```python
from build123d import *

# Parameters (mm, degrees)
SKETCH1_R           = 6.25
BOSS_EXTRUDE1_DEPTH = 4
BOSS_EXTRUDE5_START = -8
SKETCH7_R           = 8.125
SKETCH7_R_2         = 6.125
BOSS_EXTRUDE5_DEPTH = 12


with BuildPart() as part:
    # Sketch1 → Boss-Extrude1 (new body)
    with BuildSketch(Plane.XY):
        with BuildLine():
            Line((85.864132579, -9.289310318), (33.098166031, -56.8))
            Line((33.098166031, -56.8), (-33.098166031, -56.8))
            Line((-33.098166031, -56.8), (-85.864132579, -9.289310318))
            ThreePointArc((-85.864132579, -9.289310318), (-77.904361198, 12.493457969), (-68.552689408, -8.729011007))
            Line((-68.552689408, -8.729011007), (-28.491797611, -44.8))
            Line((-28.491797611, -44.8), (28.491797611, -44.8))
            Line((28.491797611, -44.8), (68.552689408, -8.729011007))
            ThreePointArc((68.552689408, -8.729011007), (77.904361198, 12.493457969), (85.864132579, -9.289310318))
        make_face()
        with Locations((-77.5, 0)):
            Circle(SKETCH1_R, mode=Mode.SUBTRACT)
        with Locations((77.5, 0)):
            Circle(SKETCH1_R, mode=Mode.SUBTRACT)
    extrude(amount=BOSS_EXTRUDE1_DEPTH)

    # Sketch7 → Boss-Extrude5 (add)
    with BuildSketch(Plane.XY.offset(4).offset(BOSS_EXTRUDE5_START)):
        with Locations((-77.5, 0)):
            Circle(SKETCH7_R)
        with Locations((-77.5, 0)):
            Circle(SKETCH7_R_2, mode=Mode.SUBTRACT)
    boss_extrude5 = extrude(amount=BOSS_EXTRUDE5_DEPTH)

    # Mirror1: Boss-Extrude5 across plane
    add(boss_extrude5.mirror(Plane(origin=(0, 0, 0), x_dir=(0, 0, 1), z_dir=(1, 0, 0))))


solid = part.part
```
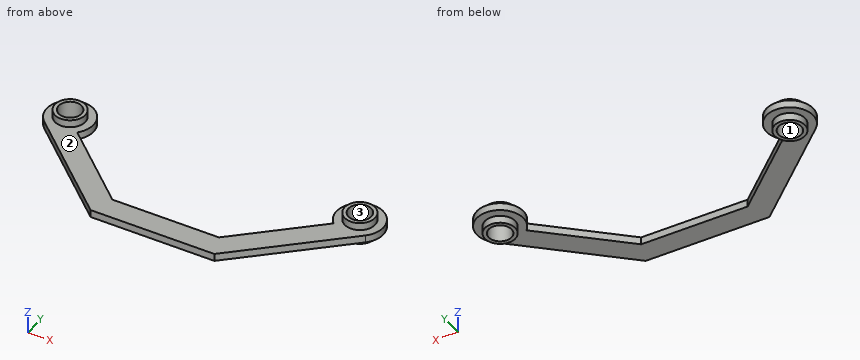
Model file for the job. Use its own axes, mm. Face numbers are marked on the shaded views. Coordinates: 2 decimals unless noted, no trailing zeros. Loops run counter-clockwise (first coordinate to the right, second up) from the corner with the lowest first, then second, coordinate; pieces in that order, holes last. Notation, with made-up numbers: (-11, -1) - (45, -1) arc R26 ccw to (45, 19) - close; hole circle Ø8 at (-36, -24.5). An arc over 180 degrees is marked (long way). Answer as a JSON object with one key per item and string values. Group by question number.
(1) Cut at B-B (y = -21.5). Give the cut face in (x, z), then the cut area to 3 significant figures.
(2) Cut at A-A (y = 0). State how many separate pieces and enclosed holes the cut face has, then the cut area to 3 significant figures.
(3) Two-plate mould, pull along Y, no slides. Class the marked faces 1, 2 and 3: released by +Y, released by -Y, zero draft, split by the parting line, or undercut.
(4) Flat gauge pins, fed straight in: pin 1 (3 mm diameter, centred on x = 35.5, z = -0.5, fed in from +Y); pin 2 (1 mm diameter, centred on x = 45, z = 1, fed in from +Y); pin 3 (3 mm diameter, centred on x = -3.5, z = 1.5, fed in from +Y). Where does each tip first touch, or does it go through?
(5) Cut at C-C (x = -77.5). Give the cut face in (y, z) (3 decimals).
(6) Probe line 1 along Y through (x, z) = (77.5, 4.5) (3 decimals); line 2 along X through (y, z) = (-2, 2.25); line 3 along Y through (x, z) = (73, -2.25). List the from-to ranges inside material, lowest first.
(7) Cut at D-D (x = -16). Give the cut face in (y, z).
Geometry says:
{
 "1": {"outline": "(-72.3, 0) - (-54.37, 0) - (-54.37, 4) - (-72.3, 4) - close; (54.37, 0) - (72.3, 0) - (72.3, 4) - (54.37, 4) - close", "area": "143 mm^2"},
 "2": {"separate pieces": "4", "enclosed holes": "0", "area": "166 mm^2"},
 "3": {"face 1": "undercut", "face 2": "zero draft", "face 3": "undercut"},
 "4": {"pin 1": "stops at y = -37.22", "pin 2": "stops at y = -29.49", "pin 3": "stops at y = -44.8"},
 "5": {"outline": "(-16.82, 0) - (-8.125, 0) - (-8.125, -4) - (-6.125, -4) - (-6.125, 8) - (-8.125, 8) - (-8.125, 4) - (-16.82, 4) - close; (6.125, -4) - (8.125, -4) - (8.125, 0) - (12.5, 0) - (12.5, 4) - (8.125, 4) - (8.125, 8) - (6.125, 8) - close"},
 "6": {"line 1": "y = -8.125 to -6.125, 6.125 to 8.125", "line 2": "x = -89.84 to -83.29, -71.71 to -65.16, 65.16 to 71.71, 83.29 to 89.84", "line 3": "y = -6.77 to -4.16, 4.16 to 6.77"},
 "7": {"outline": "(-56.8, 0) - (-44.8, 0) - (-44.8, 4) - (-56.8, 4) - close"}
}
